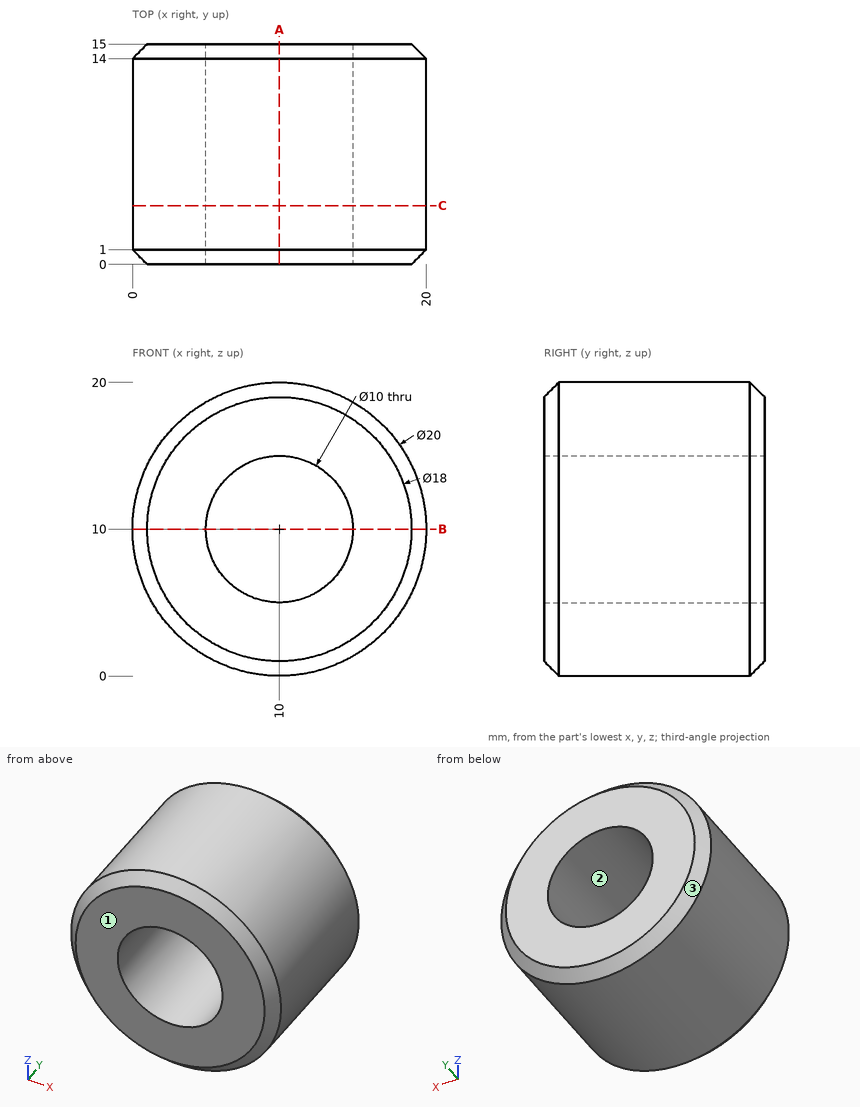
The drawing under review shows one solid part. Ordinate dimensions are in mm from its lowest x, y, z. Give positions to 0.01 mm unless a question says otherwise; leave off trailing zeros. Loops run counter-clockwise (first coordinate to the right, second up) from the corner with the lowest first, then second, coordinate; pieces in that order, holes last. Notation, with made-up numbers: M 52,31 L 77,31 A14 ccw 77,46 Z; hole C 7,18 d8. An arc over 180 degrees is marked long. One line per question, with ' | ' between items. Start each with the question number.
1. Add section B-B (z = 10). Write out the cut boundary in (x, y), plus the area to 3 significant figures.
2. To check wall thickness, follow L1, parallel to Z at x = 10, y = 7.25; L2, parallel to Z at x = 6, y = 6. State the ranges of each line that lie inside material, in increasing order.
3. The part is to be moulded in two halves that separate along Z. For the marked faces 1, 2 and 3, say which applies: released by +Z, released by -Z, zero draft, split by the parting line, or undercut.
4. Add section C-C (y = 4). Write out the cut boundary in (x, z), plus the area to 3 significant figures.
5. Insertion check: P1, Ø1.5, axis at y = 2.5, z = 15, coming from the +X side; P2, Ø2, axis at x = 7.5, y = 12, coming from the -Z side; P3, Ø8, axis at y = 13, z = 2.5, coming from the +X side. Each pin has a flat end and moves straight along its axis. Give the tip position at first contact, or say it passes through.
6. Add section A-A (x = 10). Write out the cut boundary in (y, z), plus the area to 3 significant figures.
Worked out:
1) outline: M 0,1 L 1,0 L 5,0 L 5,15 L 1,15 L 0,14 Z; M 15,0 L 19,0 L 20,1 L 20,14 L 19,15 L 15,15 Z | area: 148 mm²
2) L1: z = 0 to 5, 15 to 20 | L2: z = 0.83 to 7, 13 to 19.17
3) face 1: zero draft | face 2: undercut | face 3: split by the parting line
4) outline: C 10,10 d20; hole C 10,10 d10 | area: 236 mm²
5) P1: stops at x = 19.05 | P2: stops at z = 0.11 | P3: stops at x = 19.37
6) outline: M 0,1 L 1,0 L 14,0 L 15,1 L 15,5 L 0,5 Z; M 0,15 L 15,15 L 15,19 L 14,20 L 1,20 L 0,19 Z | area: 148 mm²
